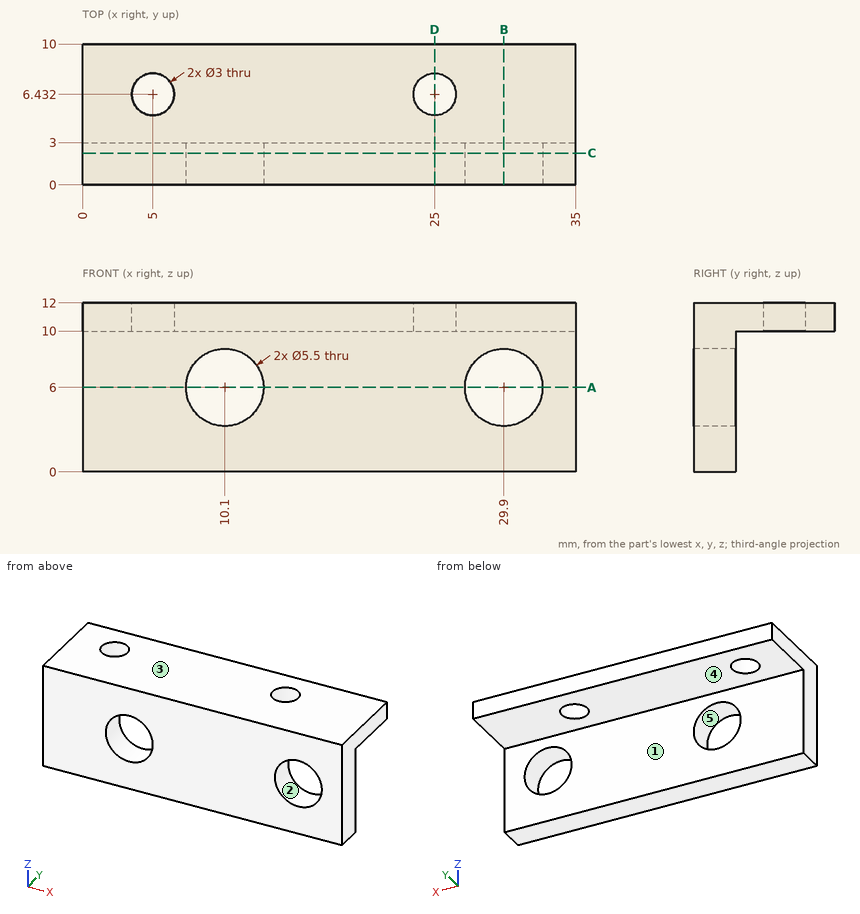
For this review, use the dimensioned drawing (mm, ordinates from the lowest corner) and the shaded views. A direction names the side the tool comes from. Give positions to 0.01 mm unless a question says otherwise; leave off trailing zeros. Order: outer loops, then holes, each group sorted by start corner. A loop starts at its lowest first (then second) coordinate and runs counter-clockwise, first axis right, second up.
1. Add section B-B, the plane x = 29.9. State the section outline as (y, z) points.
Solution:
outline: (0, 0) - (3, 0) - (3, 3.25) - (0, 3.25) - close; (0, 8.75) - (3, 8.75) - (3, 10) - (10, 10) - (10, 12) - (0, 12) - close
2. To check wall thickness, follow L1, parallel to X at y = 6.5, z = 11.25; L2, parallel to Z at x = 10.1, y = 1.35; L3, parallel to Z at x = 5.5, y = 9.25. State the ranges of each line that lie inside material, in increasing order.
Solution:
L1: x = 0 to 3.5, 6.5 to 23.5, 26.5 to 35
L2: z = 0 to 3.25, 8.75 to 12
L3: z = 10 to 12
3. Add section A-A, the plane z = 6. State the section outline as (x, y) points.
Solution:
outline: (0, 0) - (7.35, 0) - (7.35, 3) - (0, 3) - close; (12.85, 0) - (27.15, 0) - (27.15, 3) - (12.85, 3) - close; (32.65, 0) - (35, 0) - (35, 3) - (32.65, 3) - close
4. Add section D-D, the plane x = 25. State the section outline as (y, z) points.
Solution:
outline: (0, 0) - (3, 0) - (3, 10) - (4.93, 10) - (4.93, 12) - (0, 12) - close; (7.93, 10) - (10, 10) - (10, 12) - (7.93, 12) - close
5. Add section C-C, the plane y = 2.25. State the section outline as (x, z) points.
Solution:
outline: (0, 0) - (35, 0) - (35, 12) - (0, 12) - close; hole circle Ø5.5 at (10.1, 6); hole circle Ø5.5 at (29.9, 6)
6. Mouldability with a two-part tool opening along Z and no side actions: class the marked faces 1, 2 and 3 as +Z half, -Z half, draft (parallel to the pull), parting line (faces both ways), or undercut.
Solution:
face 1: draft
face 2: undercut
face 3: +Z half
7. For pin 1 Ø3.5 at (x, z) = (29.9, 6) entering from +Y; pin 2 Ø3 at (x, z) = (26.5, 4) entering from +Y; pin 3 Ø3.5 at (x, y) = (11, 6.5) entering from -Z, all flat-tipped, find the tip position at first contact; note any pin that passes through.
Solution:
pin 1: passes through
pin 2: stops at y = 3
pin 3: stops at z = 10
8. Tool access review of the marked faces 4 and 5: name each direction out of +Z, -Z, +X, -X, +Y, -Y from which nothing blocks a thin tool from reaching the whole face with its end or side.
Solution:
face 4: -Z, +X, -X, +Y
face 5: +Y, -Y
